Can you work these out from the model? Positions are in its coordinate system, mm. Coordinates: 2 decimals unless noted, no trailing zeros. Loops run counter-clockwise (first coordinate to the right, second up) from the corner with the lowest first, then second, coordinate; pieces in that order, holes last. Notation, with made-up numbers: M -20,3.5 L -4,3.5 A27 ccw -4,42.5 Z; hole C 19.5,22 d8. An arc over 180 degrees is marked long. Answer as a JSON object with one key per item and string values. Group by question number.
Item 1: If I drill on line 1 (Y direction, x = -0.05, z = 9.75); line 2 (Z direction, x = 0, y = 0); line 3 (X direction, y = 0.7, z = 0.5), over which ranges is the centre line in solid material (lowest first)?
Item 2: Suppose I cut it at C-C (z = 0.5). Write out the boundary of the cut face in (x, y) (3 decimals).
Item 3: I'm going to push flat-ended pins straight in: pin 1 Ø0.8 at (x, z) = (0.5, -6.5) entering from +Y; pin 2 Ø0.6 at (x, y) = (0.5, 0.5) entering from -Z. Where does each tip first touch, or does it pass through?
Item 4: We'd pull the mould along X, two halves only. Please class faces 1 (the cylindrical face through (0.02, -0.01, -6.75)), 2 (the flat face through (0, 0, 5)): +X half, -X half, draft (parallel to the pull), parting line (faces both ways), or undercut.
Item 5: Suppose I cut it at B-B (x = 0). Write out the boundary of the cut face in (y, z) (3 decimals).
Item 6: Suppose I cut it at A-A (z = 12.25). Write out the boundary of the cut face in (x, y) (3 decimals), then the cut area to 3 significant figures.
```python
from build123d import *

# Parameters (mm, degrees)
SKETCH1_R                = 1.025
BOSS_EXTRUDE1_DEPTH      = 12
CUT_EXTRUDE1_DEPTH       = 7
BOSS_EXTRUDE2_START      = 4
SKETCH3_R                = 1.025
BOSS_EXTRUDE2_DEPTH      = 4
SKETCH6_R                = 1.025
BOSS_EXTRUDE5_DEPTH      = 7
BOSS_EXTRUDE6_START      = 2
SKETCH7_R                = 1.025
BOSS_EXTRUDE6_DEPTH      = 2
BOSS_EXTRUDE8_DEPTH      = 0.6
BOSS_EXTRUDE8_DEPTH_BACK = 0.6


with BuildPart() as part:
    # Sketch1 → Boss-Extrude1 (new body)
    with BuildSketch(Plane.XY):
        Circle(SKETCH1_R)
    extrude(amount=BOSS_EXTRUDE1_DEPTH)

    # Sketch2 → Cut-Extrude1 (cut)
    with BuildSketch(Plane.XY.offset(12)):
        Polygon((0.866025404, 0), (0.433012702, 0.75), (-0.433012702, 0.75), (-0.866025404, 0), (-0.433012702, -0.75), (0.433012702, -0.75), align=None)
    extrude(amount=-CUT_EXTRUDE1_DEPTH, mode=Mode.SUBTRACT)

    # Sketch3 → Boss-Extrude2 (add)
    with BuildSketch(Plane(origin=(0, 0, 0), x_dir=(-1, 0, 0), z_dir=(0, 0, -1)).offset(BOSS_EXTRUDE2_START)):
        Circle(SKETCH3_R)
    extrude(amount=-BOSS_EXTRUDE2_DEPTH)

    # Sketch6 → Boss-Extrude5 (add)
    with BuildSketch(Plane.XY.offset(12)):
        with Locations(Location((0, 0, 0), (0, 0, 180))):
            Circle(SKETCH6_R)
        Polygon((0.866025404, 0), (0.433012702, 0.75), (-0.433012702, 0.75), (-0.866025404, 0), (-0.433012702, -0.75), (0.433012702, -0.75), align=None, mode=Mode.SUBTRACT)
    extrude(amount=BOSS_EXTRUDE5_DEPTH)

    # Sketch7 → Boss-Extrude6 (add)
    with BuildSketch(Plane(origin=(0, 0, -4), x_dir=(-1, 0, 0), z_dir=(0, 0, -1)).offset(BOSS_EXTRUDE6_START)):
        Circle(SKETCH7_R)
    extrude(amount=-BOSS_EXTRUDE6_DEPTH)

    # Sketch8 → Boss-Extrude8 (add, two sides: drawn at the far end of the back side and taken through both)
    with BuildSketch(Plane(origin=(0, 0, 0), x_dir=(1, 0, 0), z_dir=(0, 1, 0)).offset(-BOSS_EXTRUDE8_DEPTH_BACK)):
        with BuildLine():
            ThreePointArc((0.75, 6), (0, 6.75), (-0.75, 6))
            Line((-0.75, 6), (0.75, 6))
        make_face()
        with BuildLine():
            Line((0.75, 6), (-0.75, 6))
            ThreePointArc((-0.75, 6), (0, 5.25), (0.75, 6))
        make_face()
    extrude(amount=BOSS_EXTRUDE8_DEPTH + BOSS_EXTRUDE8_DEPTH_BACK)


solid = part.part
```
From the geometry:
{
 "1": {"line 1": "-1.02 to -0.75, 0.75 to 1.02", "line 2": "-6.75 to 5", "line 3": "-0.75 to 0.75"},
 "2": {"outline": "C 0,0 d2.05"},
 "3": {"pin 1": "y = 0.6", "pin 2": "z = -6.72"},
 "4": {"face 1": "parting line", "face 2": "undercut"},
 "5": {"outline": "M -1.025,-6 L -0.6,-6 L -0.6,-6.75 L 0.6,-6.75 L 0.6,-6 L 1.025,-6 L 1.025,19 L 0.75,19 L 0.75,5 L -0.75,5 L -0.75,19 L -1.025,19 Z"},
 "6": {"outline": "C 0,0 d2.05; hole M -0.866,0 L -0.433,-0.75 L 0.433,-0.75 L 0.866,0 L 0.433,0.75 L -0.433,0.75 Z", "area": "1.35 mm2"}
}
